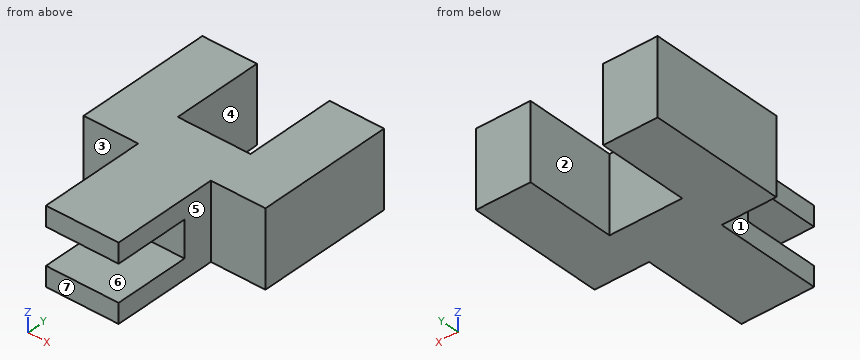
```python
from build123d import *

# Parameters (mm, degrees)
F1_DEPTH = 25
F2_W     = 25
F2_H     = 12
F3_DEPTH = 60.001


with BuildPart() as f1:
    # F0 (on Top) → F1 (new body)
    with BuildSketch(Plane.XY):
        Polygon((0, 45), (0, 0), (18, 0), (18, -35), (42, -35), (42, 0), (60, 0), (60, 45), (42, 45), (42, 15), (18, 15), (18, 45), align=None)
    extrude(amount=F1_DEPTH)

    # F2 (on Right) → F3 (cut, through all)
    with BuildSketch(Plane.YZ):
        with Locations((-22.5, 12.5)):
            Rectangle(F2_W, F2_H)
    extrude(amount=F3_DEPTH, mode=Mode.SUBTRACT)


solid = f1.part
```
Geometry: final body of the model. Coordinates: model frame, mm. Face numbers are marked on the shaded views. A direction names the side the tool comes from. Give positions to 0.01 mm unless a question says otherwise; leave off trailing zeros. Order: outer loops, then holes, each group sorted by start corner. A loop starts at its lowest first (then second) coordinate and runs counter-clockwise, first axis right, second up. Notation, with made-up numbers: (-23.75, 74) -> (-13.75, 74) arc R15 cw to (-13.75, 81) -> close; hole circle Ø8 at (11.5, -31.75). An arc over 180 degrees is marked (long way). Write each question's results on one line, items separated by ' | '. Start each with the question number.
1) Section B-B (z = 21.5). Return loops of the section in (x, y), then the cut area to 3 significant figures.
2) First-contact query: pin 1 (4 mm diameter, centred on x = 46, z = 3.5, fed in from -Y); pin 2 (6 mm diameter, centred on y = -8.5, z = 4.5, fed in from -X); pin 3 (6 mm diameter, centred on x = 37.5, z = 3.5, fed in from +Y). Flat tips, straight axial feed; report the tip coordinate or a pass-through.
3) Section C-C (x = 30.5). Return loops of the section in (y, z), then the cut area to 3 significant figures.
4) Set-up query: the marked faces 4, 5, 6 and 7. Return all of +Z, -Z, +X, -X, +Y, -Y with unobstructed straight access to the full face (end or side cutting, diameter ignored); none if empty.
5) Section D-D (y = 17). Return loops of the section in (x, z), then the cut area to 3 significant figures.
6) Draft query along X for the marked faces 1, 2 and 3. Return one class per face: pulls with the +X half, pulls with the -X half, needs draft (parallel to the pull), parting line crosses it, or undercut.
7) Line query: line 1 (X direction, y = 22.5, z = 2.5); line 2 (Z direction, x = 37, y = -17.5); line 3 (Y direction, x = 44, z = 3.5). Output: solid intervals per line, ascending. Write a range as from..to.
8) Section A-A (y = -11). Return loops of the section in (x, z), then the cut area to 3 significant figures.
Calculated:
1) outline: (0, 0) -> (18, 0) -> (18, -35) -> (42, -35) -> (42, 0) -> (60, 0) -> (60, 45) -> (42, 45) -> (42, 15) -> (18, 15) -> (18, 45) -> (0, 45) -> close | area: 2,820 mm2
2) pin 1: y = 0 | pin 2: x = 18 | pin 3: y = 15
3) outline: (-35, 0) -> (15, 0) -> (15, 25) -> (-35, 25) -> (-35, 18.5) -> (-10, 18.5) -> (-10, 6.5) -> (-35, 6.5) -> close | area: 950 mm2
4) face 4: +Z, -Z, +Y | face 5: +Z, -Z, +X, -Y | face 6: +X, -X, -Y | face 7: +Z, -Z, +X, -X, -Y
5) outline: (0, 0) -> (18, 0) -> (18, 25) -> (0, 25) -> close; (42, 0) -> (60, 0) -> (60, 25) -> (42, 25) -> close | area: 900 mm2
6) face 1: pulls with the -X half | face 2: undercut | face 3: needs draft
7) line 1: 0..18, 42..60 | line 2: 0..6.5, 18.5..25 | line 3: 0..45
8) outline: (18, 0) -> (42, 0) -> (42, 6.5) -> (18, 6.5) -> close; (18, 18.5) -> (42, 18.5) -> (42, 25) -> (18, 25) -> close | area: 312 mm2
